Verification items for the finished model (mm, model axes). Face numbers are marked on the shaded views. A direction names the side the tool comes from. Coordinates: 2 decimals unless noted, no trailing zeros. Loops run counter-clockwise (first coordinate to the right, second up) from the corner with the lowest first, then second, coordinate; pieces in that order, holes last.
Q1. Sectioned sample at B-B (y = -5). Enter the section's corners in (x, z), then the cut area to 3 significant figures.
Q2. Material ranges on probe 1 along Z at (x, y) = (32, 0); probe 2 along X at (y, z) = (19, -28.5); probe 3 along Z at (x, y) = (15, -14), recorded low to high.
Q3. Sectioned sample at C-C (z = -5). Enter the section's corners in (x, y).
Q4. Access from +Z, -Z, +X, -X, +Y, -Y to the whole of each face (thin tool, end or side, straight path). Record for the marked faces 1, 2, 3 and 4.
Q5. Go/stop test with flat-tipped pins: P1, Ø5, axis at y = 6.5, z = -16, coming from the +X side; P2, Ø12.5, axis at x = -1, z = -67.5, coming from the -Y side; P3, Ø18, axis at x = -13.5, z = -28.5, coming from the +Y side; P4, Ø12, axis at y = -1, z = -0.5, coming from the -X side. Record where each tip stops, or that it passes through.
Q6. Sectioned sample at D-D (x = 21). Enter the section's corners in (y, z).
Q7. Sectioned sample at A-A (x = -7). Enter the section's corners in (y, z).
```python
from build123d import *

# Parameters (mm, degrees)
F0_W      = 100
F0_H      = 100
F1_DEPTH  = 100
F2_W      = 21.2592259049
F2_H      = 13.5286012664
F3_DEPTH  = 20
F4_W      = 60
F4_H      = 60
F5_DEPTH  = 60
F7_W      = 35
F7_H      = 27.0690375748
F6_W      = 60
F6_H      = 60
F9_DEPTH  = 100
F10_W     = 25.1245461404
F10_H     = 22.2255568951
F12_DEPTH = 25


# Not quite as in the source:
# - a feature of the source that left no trace in its solid (it failed there, or was rolled back) is left out


with BuildPart() as f1:
    # F0 (on Top) → F1 (new body)
    with BuildSketch(Plane.XY):
        Rectangle(F0_W, F0_H)
    extrude(amount=F1_DEPTH)

    # F2 (on Top) → F3 (join)
    with BuildSketch(Plane.XY):
        Rectangle(F2_W, F2_H)
    extrude(amount=-F3_DEPTH)

    # F4 (on Top) → F5 (join)
    with BuildSketch(Plane.XY):
        Rectangle(F4_W, F4_H)
    extrude(amount=-F5_DEPTH)

    # F7 (on face) + F6 (on face) → F9 (join)
    with BuildSketch(Plane(origin=(0, 0, -60), x_dir=(1, 0, 0), z_dir=(0, 0, -1))):
        Rectangle(F7_W, F7_H)
    with BuildSketch(Plane(origin=(0, 0, -60), x_dir=(1, 0, 0), z_dir=(0, 0, -1))):
        Rectangle(F6_W, F6_H)
    extrude(amount=-F9_DEPTH)

    # F10 (on face) → F12 (join)
    with BuildSketch(Plane(origin=(0, 0, -60), x_dir=(1, 0, 0), z_dir=(0, 0, -1))):
        with Locations((0.4831599072, 0.4831608385)):
            Rectangle(F10_W, F10_H)
    extrude(amount=F12_DEPTH)


solid = f1.part
```
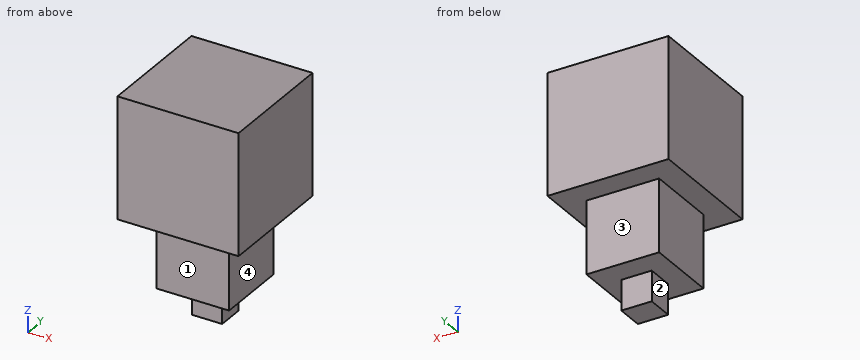
Geometry check:
1. outline: (-50, 0) - (-30, 0) - (-30, -60) - (-12.08, -60) - (-12.08, -85) - (13.05, -85) - (13.05, -60) - (30, -60) - (30, 0) - (50, 0) - (50, 100) - (-50, 100) - close
1. area: 14,200 mm2
2. probe 1: z = 0 to 100
2. probe 2: x = -30 to 30
2. probe 3: z = -60 to 100
3. outline: (-30, -30) - (30, -30) - (30, 30) - (-30, 30) - close
4. face 1: -Z, +X, -X, -Y
4. face 2: -Z, -X, +Y, -Y
4. face 3: -Z, +X, -X, +Y
4. face 4: -Z, +X, +Y, -Y
5. P1: stops at x = 30
5. P2: stops at y = -11.6
5. P3: stops at y = 30
5. P4: stops at x = -50
6. outline: (-50, 0) - (-30, 0) - (-30, -60) - (30, -60) - (30, 0) - (50, 0) - (50, 100) - (-50, 100) - close
7. outline: (-50, 0) - (-30, 0) - (-30, -60) - (-11.6, -60) - (-11.6, -85) - (10.63, -85) - (10.63, -60) - (30, -60) - (30, 0) - (50, 0) - (50, 100) - (-50, 100) - close
